Check sheet for the modelled part. Datum: model origin and axes. Units: mm. A direction names the side the tool comes from. Give positions to 0.01 mm unless a question says otherwise; leave off trailing zeros. Order: outer loops, then holes, each group sorted by start corner. A loop starts at its lowest first (then second) coordinate and runs counter-clockwise, first axis right, second up.
```python
from build123d import *

# Parameters (mm, degrees)
PAD_DEPTH    = 30
PAD001_DEPTH = 9
PAD002_DEPTH = 4.5
SKETCH003_R  = 7.5
POCKET_DEPTH = 30.001


with BuildPart() as part:
    # Sketch → Pad (new body)
    with BuildSketch(Plane.XY):
        with BuildLine():
            Line((-3.1e-05, 15), (17.999969, 15))
            Line((17.999969, 15), (17.999969, -15))
            Line((17.999969, -15), (0, -15))
            ThreePointArc((-3.1e-05, 15), (-15, -1.5e-05), (0, -15))
        make_face()
    extrude(amount=PAD_DEPTH)

    # Sketch001 → Pad001 (join)
    with BuildSketch(Plane.XY):
        Polygon((17.999969, 15), (50.999969, 15), (59.999969, 6), (59.999969, -6), (50.999969, -15), (17.999969, -15), align=None)
    extrude(amount=PAD001_DEPTH)

    # Sketch002 → Pad002 (join, symmetric)
    with BuildSketch(Plane.XZ):
        Polygon((17.999969, 30), (17.999969, 9), (59.999969, 9), align=None)
    extrude(amount=PAD002_DEPTH, both=True)

    # Sketch003 (on Face7 of Pad002) → Pocket (cut, through all)
    with BuildSketch(Plane.XY.offset(30)):
        Circle(SKETCH003_R)
    extrude(amount=-POCKET_DEPTH, mode=Mode.SUBTRACT)


solid = part.part
```
(1) Cross-section at D-D on y = 8.75. Enter the section's corners in (x, z), then the cut area to 3 significant figures.
Response values:
outline: (-12.18, 0) - (57.25, 0) - (57.25, 9) - (18, 9) - (18, 30) - (-12.18, 30) - close
area: 1,260 mm2
(2) Cross-section at C-C on x = 41.5. Enter the section's corners in (y, z), then the cut area to 3 significant figures.
Response values:
outline: (-15, 0) - (15, 0) - (15, 9) - (4.5, 9) - (4.5, 18.25) - (-4.5, 18.25) - (-4.5, 9) - (-15, 9) - close
area: 353 mm2
(3) Cross-section at A-A on y = 0. Enter the section's corners in (x, z).
Response values:
outline: (-15, 0) - (-7.5, 0) - (-7.5, 30) - (-15, 30) - close; (7.5, 0) - (60, 0) - (60, 9) - (18, 30) - (7.5, 30) - close
(4) Gauge pin test, flat ends, axial feed: pin 1 Ø5 at (x, y) = (36.5, 7.5) entering from +Z; pin 2 Ø6 at (y, z) = (-11.5, 9.5) entering from +X; pin 3 Ø8.5 at (y, z) = (-9.5, 20.5) entering from +X. Record the tip position at first contact, or that the pin passes through.
Response values:
pin 1: stops at z = 9
pin 2: stops at x = 57.46
pin 3: stops at x = 18
(5) Release check for a two-part mould opening along Y. For faces 1 (the face through (23, 0, 0)), 2 (the face through (-7.493, 0.33, 15.21)), 3 (the face through (20, -15, 8)), 4 (the face through (19, 15, 8)) record: released by +Y, released by -Y, zero draft, split by the parting line, or undercut.
Response values:
face 1: zero draft
face 2: undercut
face 3: released by -Y
face 4: released by +Y
(6) Set-up check for faces 5 (the face through (39, 10, 9)), 6 (the face through (60, 0, 4)), 7 (the face through (18, -10, 19)): record each of +Z, -Z, +X, -X, +Y, -Y from which the full face is reachable in a straight line by a thin tool's end or side.
Response values:
face 5: +Z, +X, +Y
face 6: +Z, -Z, +X, +Y, -Y
face 7: +Z, +X, -Y
(7) Material ranges on L1, parallel to Y at x = 0, z = 9.5; L2, parallel to Y at x = 44.5, z = 13.75; L3, parallel to Y at x = -5, z = 13.5, recorded low to high.
Response values:
L1: y = -15 to -7.5, 7.5 to 15
L2: y = -4.5 to 4.5
L3: y = -14.14 to -5.59, 5.59 to 14.14
(8) Cross-section at B-B on z = 5. Enter the section's corners in (x, y).
Response values:
outline: (0, -15) - (51, -15) - (60, -6) - (60, 6) - (51, 15) - (0, 15) arc R15 ccw to start; hole circle Ø15 at (0, 0)
